The listing builds one solid part. Answer for the finished solid, in the listing's coordinates (mm). Face numbers are marked on the shaded views. A direction names the side the tool comes from. Round coordinates to 2 decimals unless told otherwise and drop trailing zeros. Loops run counter-clockwise (first coordinate to the right, second up) from the corner with the lowest first, then second, coordinate; pieces in that order, holes last. Notation, with made-up numbers: (-28.5, 54.5) - (10.5, 54.5) arc R12 ccw to (10.5, 61.5) - close; hole circle Ø4 at (-15, 39). An arc over 180 degrees is marked (long way). One line per item, written item: value.
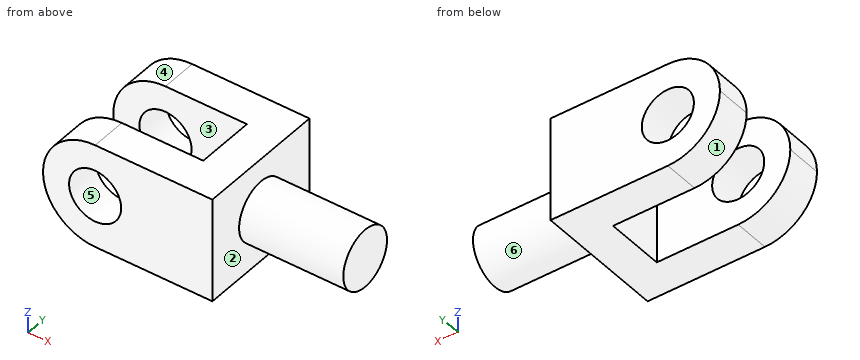
```python
from build123d import *

# Parameters (mm, degrees)
F1_DEPTH = 81.28
F2_R     = 20.32
F3_DEPTH = 101.6
F4_R     = 40.63999
F5_R     = 40.63999
F6_R     = 22.86
F7_DEPTH = 81.28


# Not quite as in the source:
# - a fillet or chamfer is up to 0.001 mm smaller than in the source, because OpenCascade refuses the exact size


with BuildPart() as f1:
    # F0 (on Top) → F1 (new body)
    with BuildSketch(Plane.XY):
        Polygon((0, -36.7104701635), (0, 0), (0, 9.0095298365), (0, 36.9495298365), (-132.08, 36.9495298365), (-132.08, 9.0095298365), (-27.94, 9.0095298365), (-27.94, -36.7104701635), (-132.08, -36.7104701635), (-132.08, -64.6504701635), (0, -64.6504701635), align=None)
    extrude(amount=F1_DEPTH)

    # F2 (on face) → F3 (cut)
    with BuildSketch(Plane.XZ.offset(64.6504701635)):
        with Locations((-91.44, 40.64)):
            Circle(F2_R)
    extrude(amount=-F3_DEPTH, mode=Mode.SUBTRACT)

    # F4 (radius 40.64 in the source; OpenCascade refuses exactly that, so slightly less here)
    f4_edges = [f1.edges().sort_by_distance(p)[0] for p in [
        (-132.08, -50.68047, 81.28),
        (-132.08, -50.68047, 0),
    ]]
    fillet(f4_edges, radius=F4_R)

    # F5 (radius 40.64 in the source; OpenCascade refuses exactly that, so slightly less here)
    f5_edges = [f1.edges().sort_by_distance(p)[0] for p in [
        (-132.08, 22.97953, 81.28),
        (-132.08, 22.97953, 0),
    ]]
    fillet(f5_edges, radius=F5_R)

    # F6 (on face) → F7 (join)
    with BuildSketch(Plane.YZ):
        with Locations((-13.8504701635, 40.64)):
            Circle(F6_R)
    extrude(amount=F7_DEPTH)


solid = f1.part
```
1) Each of these flat-tipped pins is pushed along its axis until it touches: pin 1 Ø8 at (y, z) = (-16.5, 33.5) entering from -X; pin 2 Ø6 at (y, z) = (-42.5, 59) entering from +X. Where does it stop, or does it pass through?
Final values:
pin 1: x = -27.94
pin 2: x = 0
2) A cutting plane is placed at D-D on x = -94. Give the vertices of the cut face in (y, z).
Final values:
outline: (-64.65, 0.08) - (-36.71, 0.08) - (-36.71, 20.48) - (-64.65, 20.48) - close; (-64.65, 60.8) - (-36.71, 60.8) - (-36.71, 81.2) - (-64.65, 81.2) - close; (9.01, 0.08) - (36.95, 0.08) - (36.95, 20.48) - (9.01, 20.48) - close; (9.01, 60.8) - (36.95, 60.8) - (36.95, 81.2) - (9.01, 81.2) - close
3) Consider L1, parallel to Y at x = -68, z = 53.5; L2, parallel to Z at x = -91.44, y = 26; L3, parallel to X at y = 15, z = 40. Determine where each line is inside the solid, lowest interval first.
Final values:
L1: -64.65 to -36.71, 9.01 to 36.95
L2: 0 to 20.32, 60.96 to 81.28
L3: -132.07 to -111.75, -71.13 to 0
4) A cutting plane is placed at A-A on x = -47.5. Give the vertices of the cut face in (y, z), and give its area (3 significant figures).
Final values:
outline: (-64.65, 0) - (-36.71, 0) - (-36.71, 81.28) - (-64.65, 81.28) - close; (9.01, 0) - (36.95, 0) - (36.95, 81.28) - (9.01, 81.28) - close
area: 4,540 mm2
5) A cutting plane is placed at C-C on z = 47.5. Give the vertices of the cut face in (x, y).
Final values:
outline: (-131.5, -64.65) - (-110.57, -64.65) - (-110.57, -36.71) - (-131.5, -36.71) - close; (-131.5, 9.01) - (-110.57, 9.01) - (-110.57, 36.95) - (-131.5, 36.95) - close; (-72.31, -64.65) - (0, -64.65) - (0, -35.66) - (81.28, -35.66) - (81.28, 7.96) - (0, 7.96) - (0, 36.95) - (-72.31, 36.95) - (-72.31, 9.01) - (-27.94, 9.01) - (-27.94, -36.71) - (-72.31, -36.71) - close
6) For a pull along X with two mould halves and no side action, classify the marked faces 4, 5 and 6 as released by +X, released by -X, zero draft, split by the parting line, or undercut.
Final values:
face 4: released by -X
face 5: undercut
face 6: zero draft
7) For the marked faces 1, 2 and 3, determine the directions among +Z, -Z, +X, -X, +Y, -Y from which every point of the face is accessible in a straight line to the end or side of a thin tool.
Final values:
face 1: -Z, -X, +Y, -Y
face 2: +X
face 3: +Z, -Z, -X
